Could you check a few things on this model? Use its own coordinates, in mm. A direction names the side the tool comes from. Coordinates: 2 decimals unless noted, no trailing zeros. Loops run counter-clockwise (first coordinate to the right, second up) from the corner with the lowest first, then second, coordinate; pieces in that order, holes last. Notation, with made-up numbers: (35, 48.25) - (84, 48.25) arc R19 ccw to (84, 79.25) - close; hole circle Ø3 at (12.5, 60.5). An arc over 180 degrees is marked (long way). One line per question, with ' | ' between items. Start each with the question number.
1. We'd pull the mould along X, two halves only. Please class faces 1 (the flat face through (15, 5, 7)), 2 (the cylindrical face through (18.4, 3.45, -11.93)), 3 (the flat face through (-14, 5, 0)): pulls with the +X half, pulls with the -X half, needs draft (parallel to the pull), parting line crosses it, or undercut.
2. I want a section at B-B, the plane z = 9.5. Write out the boundary of the cut face in (x, y), then the cut area to 3 significant figures.
3. I want a section at A-A, the plane y = 6. Write out the boundary of the cut face in (x, z), then the cut area to 3 significant figures.
4. I want a section at D-D, the plane x = 11.5. Write out the boundary of the cut face in (y, z), then the cut area to 3 significant figures.
5. I want a section at C-C, the plane y = 1.5. Write out the boundary of the cut face in (x, z).
6. Which directions (+Z, -Z, +X, -X, +Y, -Y) give clear straight access to the entire face, cutting with the end or side of a thin tool? Please do faces 4 (the flat face through (-12.73, 5.03, -5.76)), 5 (the flat face through (-7, 2, 0)), 6 (the flat face through (-9, 5, 9)), 7 (the flat face through (-22, 3, -1)).
7. Please list where these lines run through material, in increasing order: L1, parallel to X at y = 3.25, z = -8; L2, parallel to X at y = 2.75, z = -8; L3, parallel to Z at x = 16.5, y = 2. Write a range as [from, to].
8. I'm going to push flat-ended pins straight in: P1, Ø3, axis at x = 0, y = 0, coming from the -Z side; P2, Ø7.5, axis at x = -7.5, z = -1, coming from the +Y side; P3, Ø8, axis at x = -22.5, z = 4, coming from the +Y side; P4, Ø2, axis at x = -21, z = -1, coming from the -Y side. Where does each tip first touch, or does it pass through?
from build123d import *
from build123d.topology import SkipClean

# Parameters (mm, degrees)
SKETCH_1_W           = 50
SKETCH_1_H           = 25
EXTRUDE_1_DEPTH      = 7
EXTRUDE_2_DEPTH      = 5
SKETCH_3_R           = 1
CUT_EXTRUDE_1_DEPTH  = 37.041642582
SKETCH_5_W           = 6
SKETCH_5_H           = 25
CUT_EXTRUDE_5_DEPTH  = 31.037476592
SKETCH_6_R           = 2
CUT_EXTRUDE_6_DEPTH  = 2.5
FILLET_2_R           = 2
FILLET_3_R           = 5
SKETCH_8_R           = 1.1
CUT_EXTRUDE_9_DEPTH  = 31.037476592
CUT_EXTRUDE_4_DEPTH  = 4
SKETCH_7_W           = 16
SKETCH_7_H           = 15
CUT_EXTRUDE_7_DEPTH  = 29.814059068
SKETCH_10_R          = 3
CUT_EXTRUDE_11_DEPTH = 3
SKETCH_12_R          = 2
EXTRUDE_3_DEPTH      = 5
SKETCH_13_W          = 10
SKETCH_13_H          = 25
SKETCH_13_W_2        = 8
SKETCH_13_H_2        = 11.5
CUT_EXTRUDE_12_DEPTH = 2


with BuildPart() as part:
    # 草图1 → 凸台-拉伸1 (new body)
    with BuildSketch(Plane(origin=(0, 0, 0), x_dir=(1, 0, 0), z_dir=(0, 1, 0))):
        Rectangle(SKETCH_1_W, SKETCH_1_H)
    extrude(amount=EXTRUDE_1_DEPTH)

    # 草图2 → 凸台-拉伸2 (add)
    with BuildSketch(Plane.XY.offset(12.5)):
        with BuildLine():
            Line((-2.828427125, 0), (2.828427125, 0))
            ThreePointArc((2.828427125, 0), (0, -4), (-2.828427125, 0))
        make_face()
    extrude_2 = extrude(amount=-EXTRUDE_2_DEPTH)

    # 草图3 → 切除-拉伸1 (cut, through all)
    with BuildSketch(Plane.XY.offset(12.5)):
        Circle(SKETCH_3_R)
    cut_extrude_1 = extrude(amount=-CUT_EXTRUDE_1_DEPTH, mode=Mode.SUBTRACT)

    # 镜向1: 凸台-拉伸2, 切除-拉伸1 across plane
    with SkipClean():  # the faces are left unmerged after this step: merging them gives an invalid solid
        add(extrude_2.mirror(Plane.XY))
        add(cut_extrude_1.mirror(Plane.XY), mode=Mode.SUBTRACT)

    # 草图5 → 切除-拉伸5 (cut, through all)
    with SkipClean():  # the faces are left unmerged after this step: merging them gives an invalid solid
        with BuildSketch(Plane(origin=(0, 7, 0), x_dir=(1, 0, 0), z_dir=(0, 1, 0))):
            with Locations((22, 0)):
                Rectangle(SKETCH_5_W, SKETCH_5_H)
        extrude(amount=-CUT_EXTRUDE_5_DEPTH, mode=Mode.SUBTRACT)

    # 草图6 → 切除-拉伸6 (cut)
    with SkipClean():  # the faces are left unmerged after this step: merging them gives an invalid solid
        with BuildSketch(Plane.XY.offset(12.5)):
            Circle(SKETCH_6_R)
        extrude(amount=-CUT_EXTRUDE_6_DEPTH, mode=Mode.SUBTRACT)

    # 圆角2
    fillet_2_edges = [part.edges().sort_by_distance(p)[0] for p in [
        (19, 3.5, 12.5),
        (19, 3.5, -12.5),
        (-25, 3.5, 12.5),
        (-25, 3.5, -12.5),
    ]]
    fillet(fillet_2_edges, radius=FILLET_2_R)

    # 圆角3
    fillet_3_edges = [part.edges().sort_by_distance(p)[0] for p in [
        (2.828427125, 0, 10),
        (-2.828427125, 0, 10),
        (2.828427125, 0, -10),
        (-2.828427125, 0, -10),
    ]]
    fillet(fillet_3_edges, radius=FILLET_3_R)

    # 草图8 → 切除-拉伸9 (cut, through all)
    with SkipClean():  # the faces are left unmerged after this step: merging them gives an invalid solid
        with BuildSketch(Plane(origin=(0, 7, 0), x_dir=(1, 0, 0), z_dir=(0, 1, 0))):
            with Locations(Location((-13, 8, 0), (0, 0, 270))):
                Circle(SKETCH_8_R)
            with Locations(Location((-13, -7.5, 0), (0, 0, 270))):
                Circle(SKETCH_8_R)
            with Locations(Location((16, 8, 0), (0, 0, 270))):
                Circle(SKETCH_8_R)
            with Locations(Location((16, 0.5, 0), (0, 0, 270))):
                Circle(SKETCH_8_R)
        extrude(amount=-CUT_EXTRUDE_9_DEPTH, mode=Mode.SUBTRACT)

    # 草图4 → 切除-拉伸4 (cut)
    with SkipClean():  # the faces are left unmerged after this step: merging them gives an invalid solid
        with BuildSketch(Plane(origin=(0, 7, 0), x_dir=(1, 0, 0), z_dir=(0, 1, 0))):
            Polygon((-9, -12.5), (11, -12.5), (11, 12.5), (-9, 12.5), (-9, 6.5), (-11.5, 6.5), (-14, 5), (-14, -5), (-11.5, -6.5), (-9, -6.5), align=None)
        extrude(amount=-CUT_EXTRUDE_4_DEPTH, mode=Mode.SUBTRACT)

    # 草图7 → 切除-拉伸7 (cut, through all)
    with SkipClean():  # the faces are left unmerged after this step: merging them gives an invalid solid
        with BuildSketch(Plane(origin=(0, 3, 0), x_dir=(1, 0, 0), z_dir=(0, 1, 0))):
            with Locations((1, 0)):
                Rectangle(SKETCH_7_W, SKETCH_7_H)
        extrude(amount=-CUT_EXTRUDE_7_DEPTH, mode=Mode.SUBTRACT)

    # 草图10 → 切除-拉伸11 (cut)
    with SkipClean():  # the faces are left unmerged after this step: merging them gives an invalid solid
        with BuildSketch(Plane.XZ):
            with Locations(Location((-20, 0, 0), (0, 0, 270))):
                Circle(SKETCH_10_R)
        extrude(amount=-CUT_EXTRUDE_11_DEPTH, mode=Mode.SUBTRACT)

    # 草图12 → 凸台-拉伸3 (add)
    with SkipClean():  # the faces are left unmerged after this step: merging them gives an invalid solid
        with BuildSketch(Plane.XZ.offset(-3)):
            with Locations(Location((-20, 0, 0), (0, 0, 270))):
                Circle(SKETCH_12_R)
        extrude(amount=EXTRUDE_3_DEPTH)

    # 草图13 → 切除-拉伸12 (cut)
    with SkipClean():  # the faces are left unmerged after this step: merging them gives an invalid solid
        with BuildSketch(Plane(origin=(0, 7, 0), x_dir=(1, 0, 0), z_dir=(0, 1, 0))):
            with Locations((-20, 0)):
                Rectangle(SKETCH_13_W, SKETCH_13_H)
            with Locations((15, -6.75)):
                Rectangle(SKETCH_13_W_2, SKETCH_13_H_2)
        extrude(amount=-CUT_EXTRUDE_12_DEPTH, mode=Mode.SUBTRACT)


solid = part.part
Results are:
1) face 1: needs draft | face 2: pulls with the +X half | face 3: undercut
2) outline: (-25, 0) - (-6.93, 0) arc R5 cw to (-2.6, -2.5) arc R3 ccw to (2.6, -2.5) arc R5 cw to (6.93, 0) - (19, 0) - (19, 5) - (11, 5) - (11, 3) - (-9, 3) - (-9, 7) - (-15, 7) - (-15, 5) - (-25, 5) - close; hole circle Ø2 at (0, 0) | area: 214 mm2
3) outline: (-15, -12.5) - (-9, -12.5) - (-9, -6.5) - (-11.5, -6.5) - (-14, -5) - (-14, 5) - (-11.5, 6.5) - (-9, 6.5) - (-9, 12.5) - (-15, 12.5) - close; (11, -12.5) - (17, -12.5) arc R2 ccw to (19, -10.5) - (19, 1) - (11, 1) - close; hole circle Ø2.2 at (-13, -8); hole circle Ø2.2 at (-13, 7.5); hole circle Ø2.2 at (16, -8); hole circle Ø2.2 at (16, -0.5) | area: 181 mm2
4) outline: (0, -12.5) - (7, -12.5) - (7, 1) - (5, 1) - (5, 12.5) - (0, 12.5) - close | area: 152 mm2
5) outline: (-25, -10.5) arc R2 ccw to (-23, -12.5) - (17, -12.5) arc R2 ccw to (19, -10.5) - (19, 10.5) arc R2 ccw to (17, 12.5) - (1.32, 12.5) - (1.32, 10) - (-1.32, 10) - (-1.32, 12.5) - (-23, 12.5) arc R2 ccw to (-25, 10.5) - close; circle Ø4 at (-20, 0); hole circle Ø6 at (-20, 0); hole circle Ø2.2 at (-13, -8); hole circle Ø2.2 at (-13, 7.5); hole (-7, -7.5) - (9, -7.5) - (9, 7.5) - (-7, 7.5) - close; hole circle Ø2.2 at (16, -8); hole circle Ø2.2 at (16, -0.5)
6) face 4: +Y | face 5: +Y, -Y | face 6: +Z, -Z, +Y | face 7: -Y
7) L1: x = [-25, -14.1], [-11.9, -9], [11, 14.9], [17.1, 19] | L2: x = [-25, -14.1], [-11.9, 14.9], [17.1, 19] | L3: z = [-12.5, -8.98], [-7.02, -1.48], [0.48, 12.5]
8) P1: stops at z = -12.5 | P2: stops at y = 3 | P3: stops at y = 5 | P4: stops at y = -2
